```python
from build123d import *

# Parameters (mm, degrees)
F0_W     = 101.6
F0_H     = 50.8
F0_R     = 4.7625
F1_DEPTH = 12.7


with BuildPart() as f1:
    # F0 (on Front) → F1 (new body)
    with BuildSketch(Plane.XZ):
        with Locations((0, 76.2)):
            Rectangle(F0_W, F0_H)
        with Locations((-34.925, 85.725)):
            Circle(F0_R, mode=Mode.SUBTRACT)
        with Locations((34.925, 85.725)):
            Circle(F0_R, mode=Mode.SUBTRACT)
        with Locations((101.6, 76.2)):
            Rectangle(F0_W, F0_H)
        with Locations((127, 85.725)):
            Circle(F0_R, mode=Mode.SUBTRACT)
        with Locations((-101.6, 76.2)):
            Rectangle(F0_W, F0_H)
        with Locations((-127, 85.725)):
            Circle(F0_R, mode=Mode.SUBTRACT)
        with Locations((101.6, 25.4)):
            Rectangle(F0_W, F0_H)
        with Locations((127, 15.875)):
            Circle(F0_R, mode=Mode.SUBTRACT)
        Polygon((50.8, 0), (50.8, 50.8), (-50.8, 50.8), (-50.8, 0), (-50.8, -101.6), (50.8, -101.6), align=None)
        with Locations((-34.925, -76.2)):
            Circle(F0_R, mode=Mode.SUBTRACT)
        with Locations((34.925, -76.2)):
            Circle(F0_R, mode=Mode.SUBTRACT)
        with Locations((-101.6, 25.4)):
            Rectangle(F0_W, F0_H)
        with Locations((-127, 15.875)):
            Circle(F0_R, mode=Mode.SUBTRACT)
    extrude(amount=F1_DEPTH)


solid = f1.part
```
The model under review builds one solid part; all positions refer to its coordinate system, in mm. A direction names the side the tool comes from. Coordinates: 2 decimals unless noted, no trailing zeros. Write each loop counter-clockwise with the first axis right and the second up, starting at its lowest first coordinate (ties: lowest second). Pieces come first, ordered by that corner, then holes. Notation, with made-up numbers: (69.25, 44) - (79.25, 44) arc R23 cw to (79.25, 59) - close; hole circle Ø7 at (19.5, -22.5). An arc over 180 degrees is marked (long way). Answer in a Markdown table with one row per item. Add a question column.
Q1. Consider section B-B on x = -36. Give the boundary of the cut face in (y, z).
Q2. To check wall thickness, follow line 1 along Z through (x, y) = (-127, -4); line 2 along X through (y, z) = (-4.5, -75.5); line 3 along Z through (x, y) = (-123, -2.25). State the ranges of each line that lie inside material, in increasing order. Write a range as from..to.
Q3. For faces 1 (the face through (34.305, -6.261, 90.447)), 2 (the face through (-50.8, -6, -50)), 3 (the face through (50.8, -6, -52)), list the 3-axis set-ups (+Z, -Z, +X, -X, +Y, -Y) from which the entire face can be reached by the end or side of a thin tool; tool diameter is ignored.
Q4. Clearance check with flat-ended pins moving along their axes: pin 1 (6.5 mm diameter, centred on y = -8.5, z = -58.5, fed in from +X); pin 2 (8.5 mm diameter, centred on x = -34.925, z = 85.725, fed in from +Y); pin 3 (4 mm diameter, centred on x = -112.5, y = -6, fed in from -Z). State where each tip first meets the part, or that it passes through.
Q5. Consider section C-C on y = -2.5. Give the number of separate pieces and of enclosed holes in the cut face, then the cut area to 3 significant figures.
Q6. Consider section A-A on z = -76.2. Give the boundary of the cut face in (x, y).
Q7. Consider section D-D on x = -83. Give the boundary of the cut face in (y, z), then the cut area to 3 significant figures.
Answers below:
| question | item | result |
|---|---|---|
| 1 | outline | (-12.7, -101.6) - (0, -101.6) - (0, -80.84) - (-12.7, -80.84) - close; (-12.7, -71.56) - (0, -71.56) - (0, 81.09) - (-12.7, 81.09) - close; (-12.7, 90.36) - (0, 90.36) - (0, 101.6) - (-12.7, 101.6) - close |
| 2 | line 1 | 0..11.11, 20.64..80.96, 90.49..101.6 |
| 2 | line 2 | -50.8..-39.64, -30.21..30.21, 39.64..50.8 |
| 2 | line 3 | 0..13.29, 18.46..83.14, 88.31..101.6 |
| 3 | face 1 | +Y, -Y |
| 3 | face 2 | -Z, -X, +Y, -Y |
| 3 | face 3 | -Z, +X, +Y, -Y |
| 4 | pin 1 | x = 50.8 |
| 4 | pin 2 | through |
| 4 | pin 3 | z = 0 |
| 5 | separate pieces | 1 |
| 5 | enclosed holes | 8 |
| 5 | area | 40,700 mm² |
| 6 | outline | (-50.8, -12.7) - (-39.69, -12.7) - (-39.69, 0) - (-50.8, 0) - close; (-30.16, -12.7) - (30.16, -12.7) - (30.16, 0) - (-30.16, 0) - close; (39.69, -12.7) - (50.8, -12.7) - (50.8, 0) - (39.69, 0) - close |
| 7 | outline | (-12.7, 0) - (0, 0) - (0, 101.6) - (-12.7, 101.6) - close |
| 7 | area | 1,290 mm² |
